Verification items for the finished model (mm, model axes). A direction names the side the tool comes from. Coordinates: 2 decimals unless noted, no trailing zeros. Loops run counter-clockwise (first coordinate to the right, second up) from the corner with the lowest first, then second, coordinate; pieces in that order, holes last. Notation, with made-up numbers: (46.5, 62.25) -> (101.5, 62.25) arc R14 ccw to (101.5, 74.25) -> close; hole circle Ø5 at (-38.5, 31). An arc over 180 degrees is marked (long way). Write item = value, one per line.
Autodesk Inventor part; units mm, degrees
ref_plane "Work Plane1" through (-2.4446, 6.0882, -1.5875) normal (0, 0, -1) x (-0.239, -0.971, 0)
ref_plane "Work Plane3" through (-129.6539, 63.7298, -14.2875) normal (0, 0, -1) x (-0.5481, 0.8364, 0)
ref_plane "YZ Plane" through (0, 0, 0) normal (1, 0, 0) x (0, 1, 0)
ref_plane "Work Plane1" through (-2.4446, 6.0882, -1.5875) normal (0, 0, -1) x (-0.239, -0.971, 0)
sketch "Sketch1" plane through (-2.4446, 6.0882, -1.5875) normal (0, 0, -1) x (-0.239, -0.971, 0)
  circle A0 centre (85.725, 10.3187) radius 2.1844
  circle A1 centre (98.425, 10.3187) radius 2.1844
  circle A2 centre (73.025, 10.3187) radius 2.1844
  line L0 (73.025, 10.3187) -> (98.425, 10.3187) construction
  line L1 (73.025, 3.9687) -> (98.425, 3.9687) construction
  line L2 (98.425, 16.6687) -> (73.025, 16.6687)
  arc A3 (73.025, 16.6687) -> (66.8404, 8.879) centre (73.025, 10.3187) ccw
  arc A4 (98.425, 3.9687) -> (104.4463, 8.3022) centre (98.425, 10.3187) ccw construction
  line L3 (73.025, 3.9687) -> (63.3473, -10.8009) construction
  arc A5 (63.3473, -10.8009) -> (66.8404, 8.879) centre (42.1019, 3.1199) ccw
  line L4 (58.7003, -37.8788) -> (62.3545, -40.2732)
  line L5 (69.323, -44.8393) -> (72.9773, -47.2337)
  line L6 (63.3473, -10.8009) -> (49.5384, -31.8756)
  arc A6 (66.8404, 8.879) -> (73.025, 3.9687) centre (73.025, 10.3187) ccw construction
  arc A7 (104.4463, 8.3022) -> (98.425, 16.6687) centre (98.425, 10.3187) ccw
  line L7 (69.2168, -44.7697) -> (68.3468, -46.0975)
  line L8 (73.0835, -47.3033) -> (72.2134, -48.6311)
  line L9 (68.7818, -45.4336) -> (72.6485, -47.9672) construction
  line L10 (70.7151, -46.7004) -> (77.6756, -36.0777) construction
  line L11 (60.5274, -39.076) -> (67.0528, -29.1172) construction
  line L12 (65.2343, -24.1298) -> (61.7541, -29.4412)
  line L13 (61.7541, -29.4412) -> (68.8713, -34.1047)
  line L14 (68.8713, -34.1047) -> (72.3515, -28.7933)
  line L15 (72.3515, -28.7933) -> (65.2343, -24.1298)
  line L16 (65.2343, -24.1298) -> (68.8713, -34.1047) construction
  line L17 (61.7541, -29.4412) -> (72.3515, -28.7933) construction
  line L18 (75.857, -31.0902) -> (72.3768, -36.4016)
  line L19 (72.3768, -36.4016) -> (79.4941, -41.0651)
  line L20 (79.4941, -41.0651) -> (82.9743, -35.7537)
  line L21 (82.9743, -35.7537) -> (75.857, -31.0902)
  line L22 (75.857, -31.0902) -> (79.4941, -41.0651) construction
  line L23 (72.3768, -36.4016) -> (82.9743, -35.7537) construction
  line L24 (181.7138, -118.4821) -> (130.5502, -84.9577) construction
  line L25 (49.5384, -31.8756) -> (83.5311, -54.149)
  line L26 (83.5311, -54.149) -> (104.4463, 8.3022)
  point P0 (85.725, 10.3187)
  point P1 (58.7003, -37.8788)
  point P2 (62.3545, -40.2732)
  point P3 (72.9773, -47.2337)
  dimension "d5" = 12.7
  dimension "d6" = 25.4
  dimension "d9" = 12.7
  dimension "d11" = 12.7
  dimension "d12" = 8.509
  dimension "d13" = 8.509
  dimension "d14" = 6.35
  dimension "d15" = 6.35
  dimension "d16" = 40.64
ref_plane "Work Plane3" through (-129.6539, 63.7298, -14.2875) normal (0, 0, -1) x (-0.5481, 0.8364, 0)
extrude "Extrusion1" add sketch "Sketch1" along normal up to surface (12.7 mm away)
sketch "Sketch2" plane through (16.667, -49.633, -14.2875) normal (0.9432, 0.3323, 0) x (0, 0, 1)
  circle A0 centre (5.1816, 25.8379) radius 2.1844
  circle A1 centre (5.1816, 13.1379) radius 2.1844
  point P0 (14.2875, -52.351)
extrude "Extrusion2" cut sketch "Sketch2" against normal blind 12.7
properties part number "AngleSupport" material "Plastic, Opaque Black"
1) Release check for a two-part mould opening along X. For faces 3 (the face through (-2.19, -90.618, -7.849)), 4 (the face through (-12, -77, -1.588)), 5 (the face through (16.695, -62.666, -7.088)) record: pulls with the +X half, pulls with the -X half, needs draft (parallel to the pull), parting line crosses it, or undercut.
Ans:
face_3 = pulls with the +X half
face_4 = needs draft
face_5 = undercut
2) Sectioned sample at B-B, the plane y = -54. Record the cut outline in (x, z), plus the area to 3 significant figures.
Ans:
outline = (4.27, -14.29) -> (18.21, -14.29) -> (18.21, -1.59) -> (4.27, -1.59) -> close
area = 177 mm2
3) Material ranges on line 1 (X direction, y = -78.5, z = -5); line 2 (Y direction, x = -30, z = -2.5); line 3 (Y direction, x = -12, z = -3.5), recorded low to high.
Ans:
line_1 = -40.43 to 10.85, 17.58 to 26.84
line_2 = -92.9 to -64.54, -60.17 to -56
line_3 = -91.42 to -59.2
4) Sectioned sample at C-C, the plane x = -11.5. Record the cut outline in (y, z), plus the area to 3 significant figures.
Ans:
outline = (-91.38, -14.29) -> (-59.12, -14.29) -> (-59.12, -1.59) -> (-91.38, -1.59) -> close
area = 410 mm2
5) Tool access check on faces 1 (the face through (12.57, -73.96, -7.85)), 2 (the face through (-32.49, -56.55, -7.85)). Record the directions out of +Z, -Z, +X, -X, +Y, -Y that give a thin tool (end or side, any length) a straight path to the whole face; none if there is none.
Ans:
face_1 = +Z, -Z
face_2 = +Z, -Z, +Y
6) Depth check by flat-ended pin: pin 1 Ø4 at (y, z) = (-58, -7.5) entering from +X; pin 2 Ø7 at (x, y) = (-32.95, -74.69) entering from +Z; pin 3 Ø2 at (x, z) = (-29.5, -9.5) entering from +Y; pin 4 Ø4 at (y, z) = (-71.5, -6) entering from +X. Enter the tip coordinate at first touch or a pass-through.
Ans:
pin_1 = 20.32
pin_2 = -1.59
pin_3 = -56
pin_4 = 25.08
